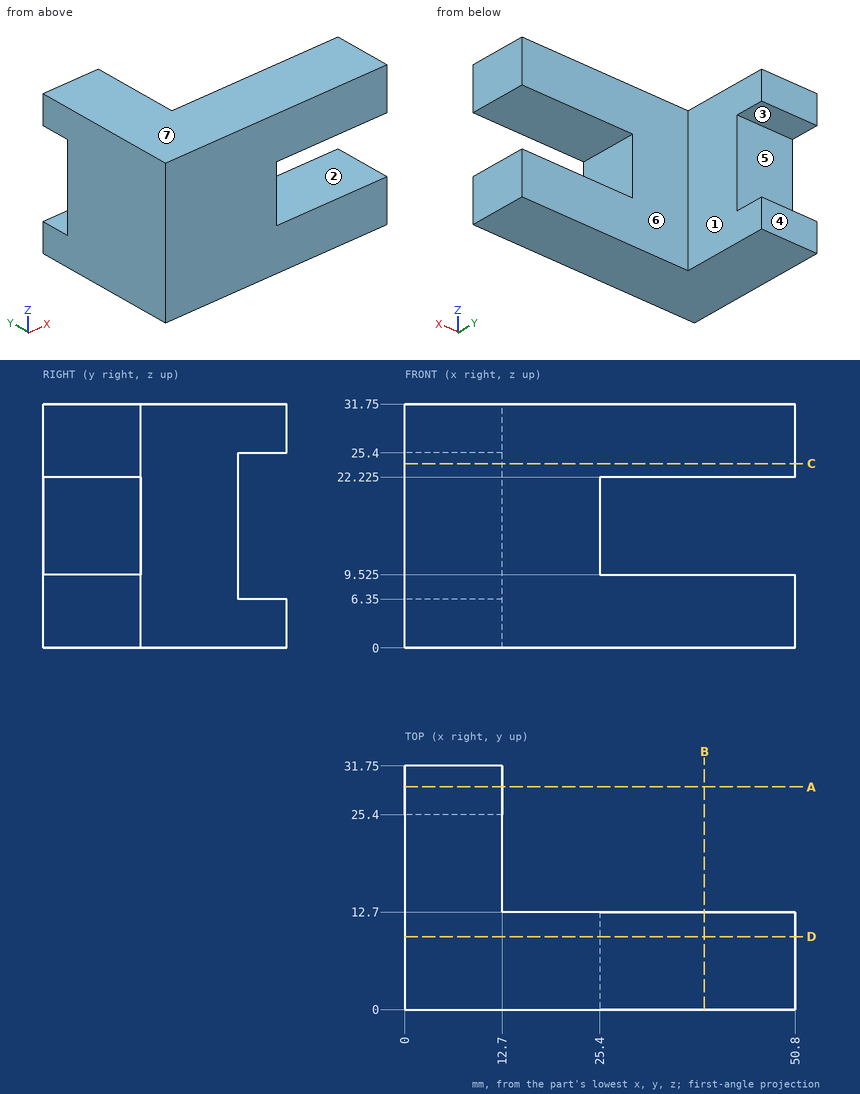
Design review of the part shown in the three views and the two pictorial views. Dimensions are in mm from the part's minimum x, y and z. A direction names the side the tool comes from. Coordinates: 2 decimals unless noted, no trailing zeros. Loops run counter-clockwise (first coordinate to the right, second up) from the corner with the lowest first, then second, coordinate; pieces in that order, holes last. Notation, with made-up numbers: (-36.75, 85) -> (-10.75, 85) arc R25 cw to (-10.75, 107) -> close; hole circle Ø10 at (76, -22.75). An arc over 180 degrees is marked (long way). Answer as CSV lines item,"result".
Item 1: Insertion check: pin 1 (10 mm diameter, centred on x = 32, y = 7, fed in from -Z); pin 2 (9.5 mm diameter, centred on x = 32, z = 18, fed in from +Y); pin 3 (1 mm diameter, centred on y = 12, z = 17.5, fed in from +X); pin 4 (5 mm diameter, centred on y = 17, z = 28.5, fed in from +X). Each pin has a flat end and moves straight along its axis. Give the tip position at first contact, or say it passes through.
Results below:
pin 1,"stops at z = 0"
pin 2,"stops at y = 12.7"
pin 3,"stops at x = 25.4"
pin 4,"stops at x = 12.7"
Item 2: Take a section at B-B, the plane x = 39. State the section outline as (y, z) points (3 decimals), and give its area (3 significant figures).
Results below:
outline,"(0, 0) -> (12.7, 0) -> (12.7, 9.525) -> (0, 9.525) -> close; (0, 22.225) -> (12.7, 22.225) -> (12.7, 31.75) -> (0, 31.75) -> close"
area,"242 mm2"
Item 3: Machinability: for the marked faces 1, 2, 3 and 4, which of the approach directions +Z, -Z, +X, -X, +Y, -Y give a long, thin tool a straight path to every point of the face, cutting with its end or side? Answer none if there is none.
Results below:
face 1,"+Z, -Z, +X, +Y"
face 2,"+X, +Y, -Y"
face 3,"+X, -X, +Y"
face 4,"+Z, -Z, +X, -X, +Y"
Item 4: Take a section at C-C, the plane z = 24. State the section outline as (x, y) points, and give its area (3 significant figures).
Results below:
outline,"(0, 0) -> (50.8, 0) -> (50.8, 12.7) -> (12.7, 12.7) -> (12.7, 25.4) -> (0, 25.4) -> close"
area,"806 mm2"
Item 5: Take a section at D-D, the plane y = 9.5. State the section outline as (x, z) points (3 decimals).
Results below:
outline,"(0, 0) -> (50.8, 0) -> (50.8, 9.525) -> (25.4, 9.525) -> (25.4, 22.225) -> (50.8, 22.225) -> (50.8, 31.75) -> (0, 31.75) -> close"
Item 6: For L1, parallel to Z at x = 12.5, y = 27; L2, parallel to Z at x = 41.5, y = 6.5 (3 decimals); L3, parallel to Y at x = 14, z = 13.5, list the stretches that pass through material, from the lowest coordinate up.
Results below:
L1,"z = 0 to 6.35, 25.4 to 31.75"
L2,"z = 0 to 9.525, 22.225 to 31.75"
L3,"y = 0 to 12.7"
Item 7: Draft analysis for pull direction Z (two halves, no side actions). For the marked faces 5, 6 and 7, state which applies: +Z half, -Z half, draft (parallel to the pull), parting line (faces both ways), or undercut.
Results below:
face 5,"undercut"
face 6,"draft"
face 7,"+Z half"
Item 8: Take a section at A-A, the plane y = 29. State the section outline as (x, z) points.
Results below:
outline,"(0, 0) -> (12.7, 0) -> (12.7, 6.35) -> (0, 6.35) -> close; (0, 25.4) -> (12.7, 25.4) -> (12.7, 31.75) -> (0, 31.75) -> close"
